CAD build for the part. Positions are in the model's coordinates, mm. A direction names the side the tool comes from. Give positions to 0.01 mm unless a question says otherwise; leave off trailing zeros. Order: outer loops, then holes, each group sorted by start corner. A loop starts at its lowest first (then second) coordinate and runs counter-clockwise, first axis right, second up.
from build123d import *

# Parameters (mm, degrees)
SKETCH1_W                    = 228.6
SKETCH1_H                    = 177.8
SKETCH1_W_2                  = 203.2
SKETCH1_H_2                  = 152.4
BOSS_EXTRUDE1_DEPTH          = 19.05
SKETCH2_W                    = 12.954
SKETCH2_H                    = 10.541
SKETCH2_W_2                  = 13.208
CUT_EXTRUDE1_DEPTH           = 8.763
SKETCH3_R                    = 2.2225
FRONT_BASE_MOUNTHOLES_DEPTH  = 7.112
FILLET2_R                    = 1.27
CHAMFER1_SIZE                = 1.27
SKETCH4_R                    = 2.2225
FRONT_BASE_MOUNTHOLES2_DEPTH = 7.62
SKETCH5_R                    = 2.2225
REAR_WALL_MOUNTHOLES_DEPTH   = 7.62
FILLET3_R                    = 1.905
SKETCH6_R                    = 2.2225
MOTOR_MOUNT_HOLES_DEPTH      = 7.366
CHAMFER2_SIZE                = 1.651
SKETCH7_R                    = 2.2225
REARBRACE_MOUNTHOLES_DEPTH   = 7.62
SKETCH8_R                    = 2.2225
SIDEBRACE_MOUNTHOLES_DEPTH   = 7.112
SKETCH9_R                    = 2.159
BATTERYMOUNT_HOLES_DEPTH     = 8.89
FILLET4_R                    = 2.54
SKETCH10_R                   = 2.2225
MOTOR_BRACE_MOUNTHOLES_DEPTH = 5.588
SKETCH11_R                   = 2.2225
DRIVETRAIN_BRACE2HOLE_DEPTH  = 7.239


with BuildPart() as part:
    # Sketch1 → Boss-Extrude1 (new body)
    with BuildSketch(Plane(origin=(0, 0, 0), x_dir=(1, 0, 0), z_dir=(0, 1, 0))):
        Rectangle(SKETCH1_W, SKETCH1_H)
        Rectangle(SKETCH1_W_2, SKETCH1_H_2, mode=Mode.SUBTRACT)
    extrude(amount=BOSS_EXTRUDE1_DEPTH)

    # Sketch2 → Cut-Extrude1 (cut)
    with BuildSketch(Plane(origin=(0, 0, -88.9), x_dir=(-1, 0, 0), z_dir=(0, 0, -1))):
        with Locations((107.823, 13.7795)):
            Rectangle(SKETCH2_W, SKETCH2_H)
        with Locations((0, 13.7795)):
            Rectangle(SKETCH2_W_2, SKETCH2_H)
        with Locations((-107.823, 13.7795)):
            Rectangle(SKETCH2_W, SKETCH2_H)
    extrude(amount=-CUT_EXTRUDE1_DEPTH, mode=Mode.SUBTRACT)

    # Sketch3 → Front-Base-MountHoles (cut)
    with BuildSketch(Plane(origin=(0, 8.509, 0), x_dir=(1, 0, 0), z_dir=(0, 1, 0))):
        with Locations(Location((-107.823, 84.5185, 0), (0, 0, 270))):
            Circle(SKETCH3_R)
        with Locations(Location((0, 84.5185, 0), (0, 0, 270))):
            Circle(SKETCH3_R)
        with Locations(Location((107.823, 84.5185, 0), (0, 0, 90))):
            Circle(SKETCH3_R)
    extrude(amount=-FRONT_BASE_MOUNTHOLES_DEPTH, mode=Mode.SUBTRACT)

    # Fillet2
    fillet2_edges = [part.edges().sort_by_distance(p)[0] for p in [
        (-107.823, 8.509, -80.137),
        (-101.346, 13.7795, -80.137),
        (-101.346, 8.509, -84.5185),
        (0, 8.509, -80.137),
        (-6.604, 8.509, -84.5185),
        (6.604, 13.7795, -80.137),
        (6.604, 8.509, -84.5185),
        (-6.604, 13.7795, -80.137),
        (101.346, 13.7795, -80.137),
        (107.823, 8.509, -80.137),
        (101.346, 8.509, -84.5185),
    ]]
    fillet(fillet2_edges, radius=FILLET2_R)

    # Chamfer1
    chamfer1_edges = [part.edges().sort_by_distance(p)[0] for p in [
        (-108.458, 8.509, -88.9),
        (101.717974388, 8.880974388, -88.9),
        (-6.232025612, 8.880974388, -88.9),
        (6.232025612, 8.880974388, -88.9),
        (-101.717974388, 8.880974388, -88.9),
        (-101.346, 14.4145, -88.9),
        (6.604, 14.4145, -88.9),
        (108.458, 8.509, -88.9),
        (101.346, 14.4145, -88.9),
        (-6.604, 14.4145, -88.9),
        (0, 8.509, -88.9),
    ]]
    chamfer(chamfer1_edges, length=CHAMFER1_SIZE)

    # Sketch4 → Front-base-MountHoles2 (cut)
    with BuildSketch(Plane(origin=(0, 0, -88.9), x_dir=(-1, 0, 0), z_dir=(0, 0, -1))):
        with Locations((-20.32, 9.525)):
            Circle(SKETCH4_R)
        with Locations((-81.28, 9.525)):
            Circle(SKETCH4_R)
        with Locations((81.28, 9.525)):
            Circle(SKETCH4_R)
        with Locations((20.32, 9.525)):
            Circle(SKETCH4_R)
    extrude(amount=-FRONT_BASE_MOUNTHOLES2_DEPTH, mode=Mode.SUBTRACT)

    # Sketch5 → Rear-Wall-MountHoles (cut)
    with BuildSketch(Plane(origin=(0, 19.05, 0), x_dir=(1, 0, 0), z_dir=(0, 1, 0))):
        with Locations(Location((-95.25, -80.772, 0), (0, 0, 270))):
            Circle(SKETCH5_R)
        with Locations(Location((-106.172, -69.85, 0), (0, 0, 270))):
            Circle(SKETCH5_R)
        with Locations(Location((106.172, -69.85, 0), (0, 0, 270))):
            Circle(SKETCH5_R)
        with Locations(Location((95.25, -80.772, 0), (0, 0, 270))):
            Circle(SKETCH5_R)
    extrude(amount=-REAR_WALL_MOUNTHOLES_DEPTH, mode=Mode.SUBTRACT)

    # Fillet3
    fillet3_edges = [part.edges().sort_by_distance(p)[0] for p in [
        (101.6, 9.525, 76.2),
        (101.6, 9.525, -76.2),
        (-101.6, 9.525, -76.2),
        (-101.6, 9.525, 76.2),
    ]]
    fillet(fillet3_edges, radius=FILLET3_R)

    # Sketch6 → Motor_Mount_Holes (cut)
    with BuildSketch(Plane(origin=(0, 19.05, 0), x_dir=(1, 0, 0), z_dir=(0, 1, 0))):
        with Locations(Location((107.95, -55.245, 0), (0, 0, 270))):
            Circle(SKETCH6_R)
        with Locations(Location((107.95, 2.54, 0), (0, 0, 270))):
            Circle(SKETCH6_R)
        with Locations(Location((107.95, 13.97, 0), (0, 0, 270))):
            Circle(SKETCH6_R)
        with Locations(Location((107.95, 25.4, 0), (0, 0, 270))):
            Circle(SKETCH6_R)
        with Locations(Location((-107.95, 25.4, 0), (0, 0, 90))):
            Circle(SKETCH6_R)
        with Locations(Location((-107.95, 13.97, 0), (0, 0, 90))):
            Circle(SKETCH6_R)
        with Locations(Location((-107.95, 2.54, 0), (0, 0, 90))):
            Circle(SKETCH6_R)
        with Locations(Location((-107.95, -55.245, 0), (0, 0, 90))):
            Circle(SKETCH6_R)
    extrude(amount=-MOTOR_MOUNT_HOLES_DEPTH, mode=Mode.SUBTRACT)

    # Chamfer2
    chamfer2_edges = [part.edges().sort_by_distance(p)[0] for p in [
        (-101.6, 19.05, 0),
        (0, 19.05, 76.2),
        (101.6, 19.05, 0),
        (0, 19.05, -76.2),
        (-101.042038418, 19.05, 75.642038418),
        (101.042038418, 19.05, 75.642038418),
        (101.042038418, 19.05, -75.642038418),
        (-101.042038418, 19.05, -75.642038418),
    ]]
    chamfer(chamfer2_edges, length=CHAMFER2_SIZE)

    # Sketch7 → RearBrace_MountHoles (cut)
    with BuildSketch(Plane(origin=(0, 19.05, 0), x_dir=(1, 0, 0), z_dir=(0, 1, 0))):
        with Locations(Location((-12.7, -82.55, 0), (0, 0, 270))):
            Circle(SKETCH7_R)
        with Locations(Location((12.7, -82.55, 0), (0, 0, 270))):
            Circle(SKETCH7_R)
    extrude(amount=-REARBRACE_MOUNTHOLES_DEPTH, mode=Mode.SUBTRACT)

    # Sketch8 → SideBrace_MountHoles (cut)
    with BuildSketch(Plane(origin=(0, 19.05, 0), x_dir=(1, 0, 0), z_dir=(0, 1, 0))):
        with Locations(Location((107.95, 73.66, 0), (0, 0, 270))):
            Circle(SKETCH8_R)
        with Locations(Location((107.95, 48.26, 0), (0, 0, 90))):
            Circle(SKETCH8_R)
        with Locations(Location((-107.95, 48.26, 0), (0, 0, 270))):
            Circle(SKETCH8_R)
        with Locations(Location((-107.95, 73.66, 0), (0, 0, 90))):
            Circle(SKETCH8_R)
    extrude(amount=-SIDEBRACE_MOUNTHOLES_DEPTH, mode=Mode.SUBTRACT)

    # Sketch9 → BatteryMount_Holes (cut)
    with BuildSketch(Plane(origin=(0, 19.05, 0), x_dir=(1, 0, 0), z_dir=(0, 1, 0))):
        with Locations(Location((-57.15, -82.55, 0), (0, 0, 270))):
            Circle(SKETCH9_R)
        with Locations(Location((57.15, -82.55, 0), (0, 0, 90))):
            Circle(SKETCH9_R)
    extrude(amount=-BATTERYMOUNT_HOLES_DEPTH, mode=Mode.SUBTRACT)

    # Fillet4
    fillet4_edges = [part.edges().sort_by_distance(p)[0] for p in [
        (-114.3, 3.6195, -88.9),
        (114.3, 3.6195, -88.9),
        (-114.3, 9.525, 88.9),
        (114.3, 9.525, 88.9),
    ]]
    fillet(fillet4_edges, radius=FILLET4_R)

    # Sketch10 → Motor-Brace-MountHoles (cut)
    with BuildSketch(Plane.XY.offset(-76.2)):
        with Locations((48.20666, 10.541)):
            Circle(SKETCH10_R)
        with Locations((67.25666, 10.541)):
            Circle(SKETCH10_R)
        with Locations(Location((-67.25666, 10.541, 0), (0, 0, 180))):
            Circle(SKETCH10_R)
        with Locations(Location((-48.20666, 10.541, 0), (0, 0, 180))):
            Circle(SKETCH10_R)
    extrude(amount=-MOTOR_BRACE_MOUNTHOLES_DEPTH, mode=Mode.SUBTRACT)

    # Sketch11 → DriveTrain-Brace2Hole (cut)
    with BuildSketch(Plane.ZY.offset(-101.6)):
        with Locations((-25.4, 10.795)):
            Circle(SKETCH11_R)
    drivetrain_brace2hole = extrude(amount=-DRIVETRAIN_BRACE2HOLE_DEPTH, mode=Mode.SUBTRACT)

    # Mirror1: DriveTrain-Brace2Hole across plane
    add(drivetrain_brace2hole.mirror(Plane(origin=(0, 0, 0), x_dir=(0, 0, 1), z_dir=(1, 0, 0))), mode=Mode.SUBTRACT)


solid = part.part
1. Mould opens along Y. For faces 1 (the cylindrical face through (-106.598, 15.419, -12.206)), 2 (the flat face through (-26, 0, 79)), 3 (the flat face through (-108, 11.684, -3)), 4 (the flat face through (48, 11, -81.788)) say: released by +Y, released by -Y, zero draft, split by the parting line, or undercut.
2. Wall check: line 1 (X direction, y = 16.75, z = 69.85); line 2 (X direction, y = 15, z = -25.4); line 3 (Z direction, x = -73, y = 1.75). Give the ranges that are in metal, low to high.
3. Saw through at A-A on z = 11.5. Give the cut face in (x, y), plus the area to 3 significant figures.
4. 3-axis set-ups, long thin cutter, end or side, ignore diameter. For faces 5 (the flat face through (81, 10, -81.28)), 6 (the flat face through (67, 11, -81.788)), 7 (the cylindrical face through (12.8, 15.29, 80.33)), 8 (the flat face through (6.604, 14, -85)): which of +Z, -Z, +X, -X, +Y, -Y reach the whole face in a straight line?
5. Pin check, flat tips, straight feed: P1, Ø1.3, axis at x = 108.5, z = -2, coming from the +Y side; P2, Ø3, axis at y = 14, z = -84.5, coming from the -X side; P3, Ø2, axis at x = 96, z = 80.5, coming from the +Y side. Stop position of each tip, or through.
Reported:
1. face 1: zero draft
1. face 2: released by -Y
1. face 3: released by +Y
1. face 4: undercut
2. line 1: x = -114.3 to -108.39, -103.95 to -101.6, 101.6 to 103.95, 108.39 to 114.3
2. line 2: x = -114.3 to -110.17, -105.73 to -101.6, 101.6 to 105.73, 110.17 to 114.3
2. line 3: z = -88.9 to -76.2, 76.2 to 88.9
3. outline: (-114.3, 0) - (-101.6, 0) - (-101.6, 17.4) - (-103.25, 19.05) - (-114.3, 19.05) - close; (101.6, 0) - (114.3, 0) - (114.3, 19.05) - (103.25, 19.05) - (101.6, 17.4) - close
3. area: 481 mm2
4. face 5: -Z
4. face 6: none
4. face 7: +Y
4. face 8: -Z, +Y
5. P1: stops at y = 11.68
5. P2: stops at x = -101.35
5. P3: stops at y = 11.43
